Work out the finished part from the listing and answer in its coordinate system (mm). Face numbers are marked on the shaded views. Coordinates: 2 decimals unless noted, no trailing zeros. Write each loop counter-clockwise with the first axis right and the second up, starting at its lowest first coordinate (ties: lowest second). Pieces come first, ordered by that corner, then holes. Notation, with made-up numbers: (11, 2) - (17, 2) arc R19 ccw to (17, 36) - close; hole circle Ø5 at (86, -32). An arc over 180 degrees is marked (long way). Use a Markdown table: item, result. Add a question column.
(1) For a pull along Y with two mould halves and no side action, classify the marked faces 1, 2, 3 and 4 as released by +Y, released by -Y, zero draft, split by the parting line, or undercut.
(2) The part is cut by section B-B, the plane y = 0. Give the vertices of the cut face in (x, z) (3 decimals).
(3) The part is cut by section A-A, the plane x = 0. Give the vertices of the cut face in (y, z) (3 decimals), then the cut area to 3 significant figures.
(4) The part is cut by section D-D, the plane z = 7.5. State how many separate pieces and enclosed holes the cut face has, then the cut area to 3 significant figures.
(5) Given pin 1 Ø9 at (x, y) = (0, 0) entering from -Z; pin 2 Ø3 at (x, y) = (-1.5, 1) entering from +Z; pin 3 Ø3.5 at (x, y) = (0, 0) entering from +Z, each flat-ended and moving along its own axis, determine where each tip first touches the part or whether it passes through.
(6) Find the intervals of material crossed by line 1 (Y direction, x = 4.5, z = 6.5); line 2 (Y direction, x = 0, z = 8.1); line 3 (Y direction, x = 0, z = 2.25) (3 decimals), in increasing order. Write a range as from..to.
(7) The part is cut by section C-C, the plane x = -4.5. Give the vertices of the cut face in (y, z).
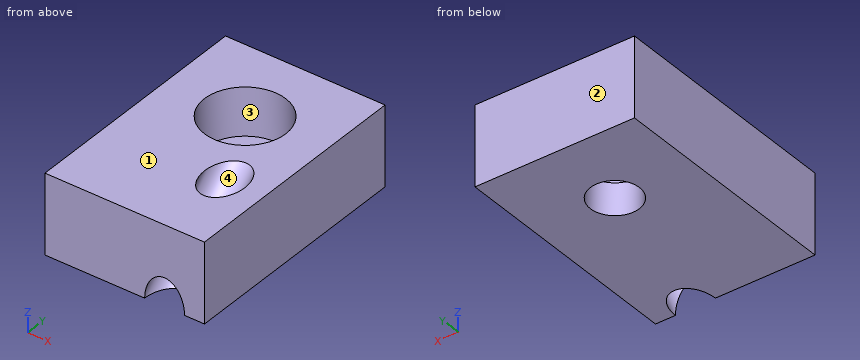
from build123d import *

# Parameters (mm, degrees)
F0_W     = 20
F0_H     = 30
F0_R     = 3.075
F1_DEPTH = 10
F2_R     = 5.1
F2_R_2   = 3.075
F3_DEPTH = 6
F5_R     = 2.5
F6_DEPTH = 25


with BuildPart() as f1:
    # F0 (on Top) → F1 (new body)
    with BuildSketch(Plane.XY):
        with Locations((0, -5)):
            Rectangle(F0_W, F0_H)
        Circle(F0_R, mode=Mode.SUBTRACT)
    extrude(amount=F1_DEPTH)

    # F2 (on face) → F3 (cut)
    with BuildSketch(Plane.XY.offset(10)):
        Circle(F2_R)
        Circle(F2_R_2, mode=Mode.SUBTRACT)
    extrude(amount=-F3_DEPTH, mode=Mode.SUBTRACT)

    # F5 (on face) → F6 (cut)
    with BuildSketch(Plane(origin=(0, -10, -10), x_dir=(-1, 0, 0), z_dir=(0, 0.707107, 0.707107))):
        with Locations((-5, 14.142136)):
            Circle(F5_R)
    extrude(amount=F6_DEPTH, mode=Mode.SUBTRACT)


solid = f1.part
Model answer:
| question | item | result |
|---|---|---|
| 1 | face 1 | zero draft |
| 1 | face 2 | released by +Y |
| 1 | face 3 | undercut |
| 1 | face 4 | undercut |
| 2 | outline | (-10, 0) - (-3.075, 0) - (-3.075, 4) - (-5.1, 4) - (-5.1, 10) - (-10, 10) - close; (3.075, 0) - (10, 0) - (10, 10) - (5.1, 10) - (5.1, 4) - (3.075, 4) - close |
| 3 | outline | (-20, 0) - (-3.075, 0) - (-3.075, 4) - (-5.1, 4) - (-5.1, 10) - (-20, 10) - close; (3.075, 0) - (10, 0) - (10, 10) - (5.1, 10) - (5.1, 4) - (3.075, 4) - close |
| 3 | area | 214 mm^2 |
| 4 | separate pieces | 1 |
| 4 | enclosed holes | 2 |
| 4 | area | 491 mm^2 |
| 5 | pin 1 | z = 0 |
| 5 | pin 2 | z = 4 |
| 5 | pin 3 | through |
| 6 | line 1 | -20..-16.96, -10.04..-2.4, 2.4..10 |
| 6 | line 2 | -20..-5.1, 5.1..10 |
| 6 | line 3 | -20..-3.075, 3.075..10 |
| 7 | outline | (-20, 0) - (10, 0) - (10, 10) - (2.4, 10) - (2.4, 4) - (-2.4, 4) - (-2.4, 10) - (-20, 10) - close |
